from build123d import *

# Parameters (mm, degrees)
F0_W     = 6.35
F0_H     = 50.8
F1_ANGLE = 180
F2_R     = 2.54
F3_DEPTH = 25.4
F4_SIZE  = 2.54


with BuildPart() as f1:
    # F0 (on Front) → F1 (revolve)
    with BuildSketch(Plane.XZ):
        with Locations((20.828, 25.4)):
            Rectangle(F0_W, F0_H)
    revolve(axis=Axis((0, 0, 25.4), (0, 0, 1)), revolution_arc=F1_ANGLE)

    # F2 (on face) → F3 (join)
    with BuildSketch(Plane(origin=(0, 0, 0), x_dir=(1, 0, 0), z_dir=(0, 0, -1))):
        with BuildLine():
            Line((43.053, 0), (24.003, 0))
            ThreePointArc((24.003, 0), (22.359215, -8.729807), (17.653, -16.263936))
            Line((17.653, -16.263936), (17.653, -25.4))
            Line((17.653, -25.4), (43.053, -25.4))
            Line((43.053, -25.4), (43.053, 0))
        make_face()
        with Locations((30.353, -12.7)):
            Circle(F2_R, mode=Mode.SUBTRACT)
        with BuildLine():
            Line((-17.653, -25.4), (-17.653, -16.263936))
            ThreePointArc((-17.653, -16.263936), (-22.359215, -8.729807), (-24.003, 0))
            Line((-24.003, 0), (-43.053, 0))
            Line((-43.053, 0), (-43.053, -25.4))
            Line((-43.053, -25.4), (-17.653, -25.4))
        make_face()
        with Locations((-30.353, -12.7)):
            Circle(F2_R, mode=Mode.SUBTRACT)
    extrude(amount=-F3_DEPTH)

    # F4
    f4_edges = [f1.edges().sort_by_distance(p)[0] for p in [
        (-32.893, 12.7, 25.4),
        (27.813, 12.7, 25.4),
    ]]
    chamfer(f4_edges, length=F4_SIZE)


solid = f1.part
Check sheet for the modelled part. Datum: model origin and axes. Units: mm. A direction names the side the tool comes from. Round coordinates to 2 decimals unless told otherwise and drop trailing zeros. Write each loop counter-clockwise with the first axis right and the second up, starting at its lowest first coordinate (ties: lowest second). Pieces come first, ordered by that corner, then holes. Notation, with made-up numbers: (68.5, 72.25) - (77.5, 72.25) arc R19 cw to (77.5, 100.25) - close; hole circle Ø8 at (12.25, -13). An arc over 180 degrees is marked (long way). Return JSON: item names as keys, results as strings.
Q1. Scan lines: L1, parallel to X at y = 12.7, z = 6; L2, parallel to Z at x = -19.5, y = 22.75; L3, parallel to X at y = 2.5, z = 29.5. Record each from-to range of solid material in increasing order. Write a range as from..to.
Returned:
{"L1": "x = -43.05..-32.89, -27.81..-12.26, 12.26..27.81, 32.89..43.05", "L2": "z = 0..25.4", "L3": "x = -23.87..-17.48, 17.48..23.87"}
Q2. Cross-section at B-B (y = 21.5). Record the boundary of the cut face in (x, z), then the cut area to 3 significant figures.
Returned:
{"outline": "(-43.05, 0) - (-17.65, 0) - (-17.65, 25.4) - (-43.05, 25.4) - close; (-10.67, 0) - (10.67, 0) - (10.67, 50.8) - (-10.67, 50.8) - close; (17.65, 0) - (43.05, 0) - (43.05, 25.4) - (17.65, 25.4) - close", "area": "2,370 mm²"}
Q3. Depth check by flat-ended pin: P1, Ø12, axis at x = -30.5, y = 3, coming from the +Z side; P2, Ø6, axis at x = -30.353, y = 12.7, coming from the -Z side; P3, Ø3, axis at y = 13.5, z = 42.5, coming from the -X side; P4, Ø6.5, axis at x = 30.353, y = 12.7, coming from the +Z side. Enter the tip coordinate at first touch or a pass-through.
Returned:
{"P1": "stops at z = 25.4", "P2": "stops at z = 0", "P3": "stops at x = -20.79", "P4": "stops at z = 23.57"}
Q4. Cross-section at A-A (z = 22). Record the boundary of the cut face in (x, y), then the cut area to 3 significant figures.
Returned:
{"outline": "(-43.05, 0) - (-17.65, 0) arc R17.65 cw to (17.65, 0) - (43.05, 0) - (43.05, 25.4) - (17.65, 25.4) - (17.65, 16.26) arc R24 ccw to (-17.65, 16.26) - (-17.65, 25.4) - (-43.05, 25.4) - close; hole circle Ø5.08 at (-30.35, 12.7); hole circle Ø5.08 at (30.35, 12.7)", "area": "1,520 mm²"}
Q5. Draft check along Y on faces 1 (the conical face through (32.93, 11.89, 23.02)), 2 (the flat face through (36, 13, 25.4)), 3 (the flat face through (30, 25.4, 13)). Enter one of: released by +Y, released by -Y, zero draft, split by the parting line, or undercut.
Returned:
{"face 1": "undercut", "face 2": "zero draft", "face 3": "released by +Y"}
Q6. Cross-section at D-D (y = 12.7). Record the boundary of the cut face in (x, z), then the cut area to 3 significant figures.
Returned:
{"outline": "(-43.05, 0) - (-32.89, 0) - (-32.89, 22.86) - (-35.43, 25.4) - (-43.05, 25.4) - close; (-27.81, 0) - (-12.26, 0) - (-12.26, 50.8) - (-20.37, 50.8) - (-20.37, 25.4) - (-25.27, 25.4) - (-27.81, 22.86) - close; (12.26, 0) - (27.81, 0) - (27.81, 22.86) - (25.27, 25.4) - (20.37, 25.4) - (20.37, 50.8) - (12.26, 50.8) - close; (32.89, 0) - (43.05, 0) - (43.05, 25.4) - (35.43, 25.4) - (32.89, 22.86) - close", "area": "1,710 mm²"}
Q7. Cross-section at C-C (y = 5.75). Record the boundary of the cut face in (x, z).
Returned:
{"outline": "(-43.05, 0) - (-16.69, 0) - (-16.69, 50.8) - (-23.3, 50.8) - (-23.3, 25.4) - (-43.05, 25.4) - close; (16.69, 0) - (43.05, 0) - (43.05, 25.4) - (23.3, 25.4) - (23.3, 50.8) - (16.69, 50.8) - close"}
Q8. Access from +Z, -Z, +X, -X, +Y, -Y to the whole of each face (thin tool, end or side, straight path). Record for faces 4 (the flat face through (-17.653, 21, 13)), 5 (the flat face through (-36, 13, 25.4)), 6 (the flat face through (-1, 18, 0)).
Returned:
{"face 4": "+Z, -Z, +Y", "face 5": "+Z, -X, +Y", "face 6": "-Z, +X, -X, +Y, -Y"}
